Input: part model. Units: mm. Frame: model coordinates. A direction names the side the tool comes from. Coordinates: 2 decimals unless noted, no trailing zeros. Order: outer loops, then holes, each group sorted by start corner. A loop starts at its lowest first (then second) coordinate and runs counter-clockwise, first axis right, second up. Notation, with made-up numbers: (-13, -39.5) -> (40, -39.5) arc R22 cw to (40, -2.5) -> close; hole circle Ø10 at (-8.75, 20). An arc over 180 degrees is marked (long way). Use one line per item in the form item = value. Start each with the question number.
1) Section query A-A on x = 0. Output: boundary loops of the cut face in (y, z) (3 decimals), then the cut area to 3 significant figures.
2) Section query B-B on y = 19. Output: boundary loops of the cut face in (x, z) (3 decimals).
3) Draft query along Z for faces 6 (the flat face through (11.176, -3, -10)), 7 (the flat face through (-23, -13, -3.937)), 8 (the flat face through (8, -3, -16.637)). Return one class per face: pulls with the +Z half, pulls with the -Z half, needs draft (parallel to the pull), parting line crosses it, or undercut.
4) Section query D-D on z = 23. Output: boundary loops of the cut face in (x, y).
5) Access query for faces 1 (the flat face through (8, 7.112, 23)), 2 (the flat face through (8, -3, -21.463)), 3 (the flat face through (-11.176, 0, -32)), 4 (the flat face through (-5.588, -3, -19)), 5 (the flat face through (23, -13, -3.937)). Directions: +Z, -Z, +X, -X, +Y, -Y. A direction counts if a zero-diameter tool reaches every point of the face in a straight line with its end or side. Return the directions, or none.
6) Ray query, line 1 along Z through (x, y) = (0, -14.5); line 2 along Z through (x, y) = (-23.5, 6); line 3 along X through (y, z) = (-4, -34.5). Return the intervals inside material, ascending.
7) Section query C-C on y = -1.5. Output: boundary loops of the cut face in (x, z) (3 decimals), then the cut area to 3 significant figures.
8) Pin query (flat end, axial travel): pin 1 (14 mm diameter, centred on y = -13, z = -11, fed in from -X); pin 2 (24.5 mm diameter, centred on x = 2, z = 13.5, fed in from +Y); pin 3 (2.5 mm diameter, centred on y = 8.5, z = -18.5, fed in from +X). Return the tip coordinate at first contact, or that it passes through.
from build123d import *

# Parameters (mm, degrees)
F0_W          = 65.024
F0_H          = 84.074
F1_DEPTH      = 35.052
F1_DEPTH_BACK = 35.052
F2_W          = 5.588
F2_H          = 4.826
F3_DEPTH      = 65.025
F4_W          = 56.330337
F4_H          = 68.819438
F5_DEPTH      = 101.6
F7_DEPTH      = 46.229
F9_DEPTH      = 254
F11_DEPTH     = 25.4
F12_DEPTH     = 65.025


with BuildPart() as f1:
    # F0 (on Right) → F1 (new body, two sides)
    with BuildSketch(Plane.YZ) as f1_sk:
        Rectangle(F0_W, F0_H)
    extrude(amount=F1_DEPTH)
    extrude(f1_sk.sketch, amount=-F1_DEPTH_BACK)

    # F2 (on face) → F3 (cut, through all)
    with BuildSketch(Plane.XZ.offset(32.512)):
        Polygon((-11.176, -16.637), (-11.176, -3.937), (-74.27659, -3.937), (-74.27659, -51.014846), (-11.176, -51.014846), (-11.176, -21.463), (-5.588, -21.463), (-5.588, -16.637), align=None)
        Polygon((76.810068, -3.937), (11.176, -3.937), (11.176, -16.637), (11.176, -21.463), (11.176, -65.525395), (76.810068, -65.525395), align=None)
        with Locations((8.382, -19.05)):
            Rectangle(F2_W, F2_H)
    extrude(amount=-F3_DEPTH, mode=Mode.SUBTRACT)

    # F4 (on face) → F5 (cut, symmetric)
    with BuildSketch(Plane.YZ.offset(35.052)):
        with Locations((35.277168, 27.424719)):
            Rectangle(F4_W, F4_H)
    extrude(amount=F5_DEPTH, both=True, mode=Mode.SUBTRACT)

    # F6 (on face) → F7 (cut, through all)
    with BuildSketch(Plane.YZ.offset(11.176)):
        Polygon((22.86, 0), (32.512, -42.037), (45.35326, -62.610321), (51.058073, 0), align=None)
    extrude(amount=-F7_DEPTH, mode=Mode.SUBTRACT)

    # F8 (on Right) → F9 (cut, symmetric)
    with BuildSketch(Plane.YZ):
        with BuildLine():
            ThreePointArc((-27.93964, 15.271957), (-17.603329, 39.968487), (7.151257, 50.164978))
            Line((7.151257, 50.164978), (-49.631871, 54.338343))
            Line((-49.631871, 54.338343), (-51.628556, 15.271957))
            Line((-51.628556, 15.271957), (-27.93964, 15.271957))
        make_face()
    extrude(amount=F9_DEPTH, both=True, mode=Mode.SUBTRACT)

    # F10 (on face) → F11 (join)
    with BuildSketch(Plane.XZ.offset(32.512)):
        with BuildLine():
            Line((9.525, 15.271957), (12.7, 15.271957))
            ThreePointArc((12.7, 15.271957), (0, 27.971957), (-12.7, 15.271957))
            Line((-12.7, 15.271957), (-9.525, 15.271957))
            ThreePointArc((-9.525, 15.271957), (0, 24.796957), (9.525, 15.271957))
        make_face()
        with BuildLine():
            ThreePointArc((-12.7, 15.271957), (0, 2.571957), (12.7, 15.271957))
            Line((12.7, 15.271957), (9.525, 15.271957))
            ThreePointArc((9.525, 15.271957), (0, 5.746957), (-9.525, 15.271957))
            Line((-9.525, 15.271957), (-12.7, 15.271957))
        make_face()
    extrude(amount=-F11_DEPTH)

    # F10 (on face) → F12 (cut, through all)
    with BuildSketch(Plane.XZ.offset(32.512)):
        with BuildLine():
            Line((-9.525, 15.271957), (9.525, 15.271957))
            ThreePointArc((9.525, 15.271957), (0, 24.796957), (-9.525, 15.271957))
        make_face()
        with BuildLine():
            ThreePointArc((-9.525, 15.271957), (0, 5.746957), (9.525, 15.271957))
            Line((9.525, 15.271957), (-9.525, 15.271957))
        make_face()
    extrude(amount=-F12_DEPTH, mode=Mode.SUBTRACT)


solid = f1.part
Answers below:
q1.outline = (-32.512, -42.037) -> (32.512, -42.037) -> (24.464, -6.985) -> (7.112, -6.985) -> (7.112, 5.747) -> (-32.512, 5.747) -> close; (-32.512, 24.797) -> (7.112, 24.797) -> (7.112, 42.037) -> (-15.332, 42.037) arc R35.052 ccw to (-25.496, 27.972) -> (-32.512, 27.972) -> close
q1.area = 3,170 mm^2
q2.outline = (-11.176, -42.037) -> (11.176, -42.037) -> (11.176, -21.463) -> (5.588, -21.463) -> (5.588, -16.637) -> (11.176, -16.637) -> (11.176, -6.985) -> (-11.176, -6.985) -> (-11.176, -16.637) -> (-5.588, -16.637) -> (-5.588, -21.463) -> (-11.176, -21.463) -> close
q3.face_6 = needs draft
q3.face_7 = pulls with the -Z half
q3.face_8 = undercut
q4.outline = (-35.05, -27.04) -> (-10.08, -27.04) -> (-10.08, -32.51) -> (-5.57, -32.51) -> (-5.57, 7.11) -> (-35.05, 7.11) -> close; (5.57, -32.51) -> (10.08, -32.51) -> (10.08, -27.04) -> (35.05, -27.04) -> (35.05, 7.11) -> (5.57, 7.11) -> close
q5.face_1 = +Z, +X, -X, +Y
q5.face_2 = +X, +Y, -Y
q5.face_3 = -Z, -X, +Y, -Y
q5.face_4 = -X, +Y, -Y
q5.face_5 = -Z, +X, +Y, -Y
q6.line_1 = -42.04 to 5.75, 24.8 to 42.04
q6.line_2 = -3.94 to 42.04
q6.line_3 = -11.18 to 11.18
q7.outline = (-35.052, -3.937) -> (-11.176, -3.937) -> (-11.176, -16.637) -> (-5.588, -16.637) -> (-5.588, -21.463) -> (-11.176, -21.463) -> (-11.176, -42.037) -> (11.176, -42.037) -> (11.176, -21.463) -> (5.588, -21.463) -> (5.588, -16.637) -> (11.176, -16.637) -> (11.176, -3.937) -> (35.052, -3.937) -> (35.052, 42.037) -> (-35.052, 42.037) -> close; hole circle Ø19.05 at (0, 15.272)
q7.area = 3,740 mm^2
q8.pin_1 = -11.18
q8.pin_2 = 7.11
q8.pin_3 = 5.59
